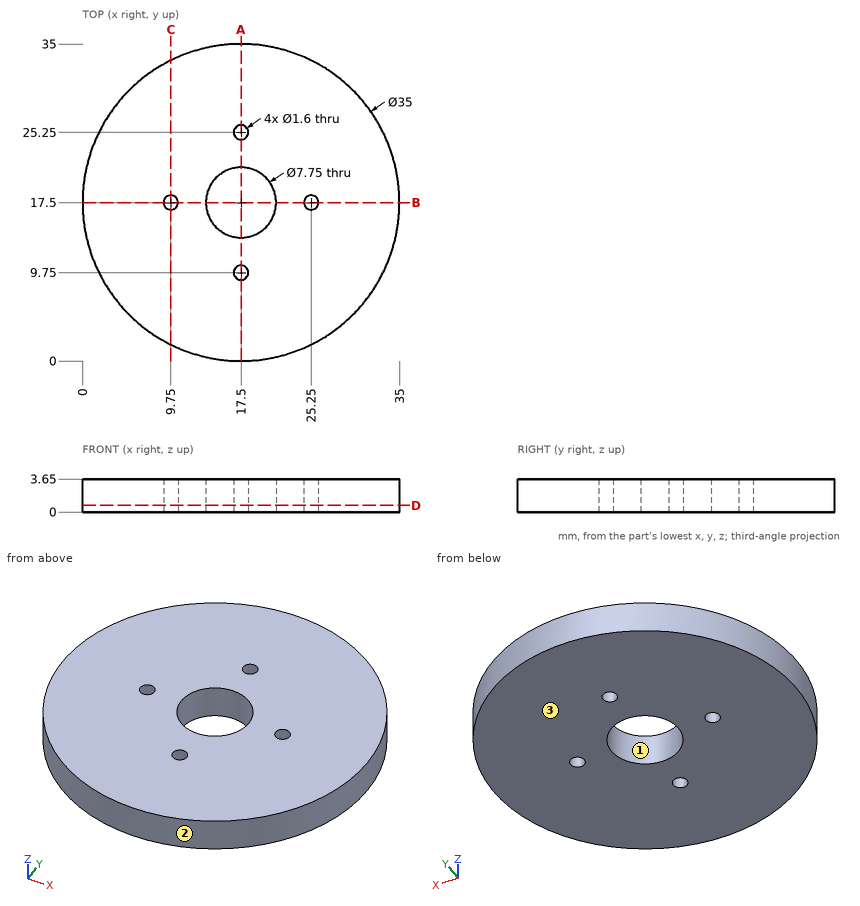
Drawing for the job (mm, zero at the part's lowest x, y, z). Give positions to 0.01 mm unless a question says otherwise; leave off trailing zeros. Loops run counter-clockwise (first coordinate to the right, second up) from the corner with the lowest first, then second, coordinate; pieces in that order, holes last.
Item 1: Mould opens along Y. For the marked faces 1, 2 and 3 say: +Y half, -Y half, draft (parallel to the pull), parting line (faces both ways), or undercut.
Check values:
face 1: undercut
face 2: parting line
face 3: draft
Item 2: Slice it at D-D (z = 0.75). Write the cut outline in (x, y) (3 decimals), plus the area to 3 significant figures.
Check values:
outline: circle Ø35 at (17.5, 17.5); hole circle Ø1.6 at (9.75, 17.5); hole circle Ø7.75 at (17.5, 17.5); hole circle Ø1.6 at (17.5, 9.75); hole circle Ø1.6 at (17.5, 25.25); hole circle Ø1.6 at (25.25, 17.5)
area: 907 mm2
Item 3: Slice it at C-C (x = 9.75). Write the cut outline in (y, z).
Check values:
outline: (1.81, 0) - (16.7, 0) - (16.7, 3.65) - (1.81, 3.65) - close; (18.3, 0) - (33.19, 0) - (33.19, 3.65) - (18.3, 3.65) - close
Item 4: Slice it at A-A (x = 17.5). Write the cut outline in (y, z) (3 decimals).
Check values:
outline: (0, 0) - (8.95, 0) - (8.95, 3.65) - (0, 3.65) - close; (10.55, 0) - (13.625, 0) - (13.625, 3.65) - (10.55, 3.65) - close; (21.375, 0) - (24.45, 0) - (24.45, 3.65) - (21.375, 3.65) - close; (26.05, 0) - (35, 0) - (35, 3.65) - (26.05, 3.65) - close
Item 5: Drop flat-ended pins along their axis: P1, Ø1.5, axis at x = 14.5, z = 1.5, coming from the +Y side; P2, Ø1.5, axis at y = 8.5, z = 2, coming from the +X side. Give the stop position or say it passes through.
Check values:
P1: stops at y = 34.85
P2: stops at x = 32.93
Item 6: Drill centre lines: line 1 along Y through (x, z) = (9.75, 1); line 2 along X through (y, z) = (16.5, 0.5); line 3 along Y through (x, z) = (20, 3.15). Where is each one in solid material? Low to high.
Check values:
line 1: y = 1.81 to 16.7, 18.3 to 33.19
line 2: x = 0.03 to 13.76, 21.24 to 34.97
line 3: y = 0.18 to 14.54, 20.46 to 34.82
